Geometry check sheet. Reference: drawing and pictorial views, mm from the part's lowest x, y, z. A direction names the side the tool comes from. Round coordinates to 2 decimals unless told otherwise and drop trailing zeros. Order: outer loops, then holes, each group sorted by start corner. A loop starts at its lowest first (then second) coordinate and runs counter-clockwise, first axis right, second up. Notation, with made-up numbers: (77, 52) -> (105, 52) arc R16 cw to (105, 69) -> close; hole circle Ø5 at (-15, -11.5). An arc over 180 degrees is marked (long way). Return JSON: item names as keys, results as strings. Group by question number.
1) Draft check along Z on the marked faces 1, 2, 3 and 4. Enter one of: pulls with the +Z half, pulls with the -Z half, needs draft (parallel to the pull), parting line crosses it, or undercut.
2) Tool access check on the marked faces 5 and 6. Record the directions out of +Z, -Z, +X, -X, +Y, -Y that give a thin tool (end or side, any length) a straight path to the whole face; none if there is none.
3) Depth check by flat-ended pin: pin 1 (5 mm diameter, centred on x = 31, z = 24.5, fed in from +Y). Enter the tip coordinate at first touch or a pass-through.
4) Section check A-A on y = 22.25. Enter the section's corners in (x, z).
5) Section check C-C on z = 17. Enter the section's corners in (x, y), plus the area to 3 significant figures.
6) Section check B-B on x = 29. Enter the section's corners in (y, z).
7) Section check D-D on x = 12.5. Enter the section's corners in (y, z), plus the area to 3 significant figures.
8) Scan lines: L1, parallel to Z at x = 35, y = 5.75; L2, parallel to X at y = 21, z = 30; L3, parallel to Y at x = 31, z = 14. Record each from-to range of solid material in increasing order.
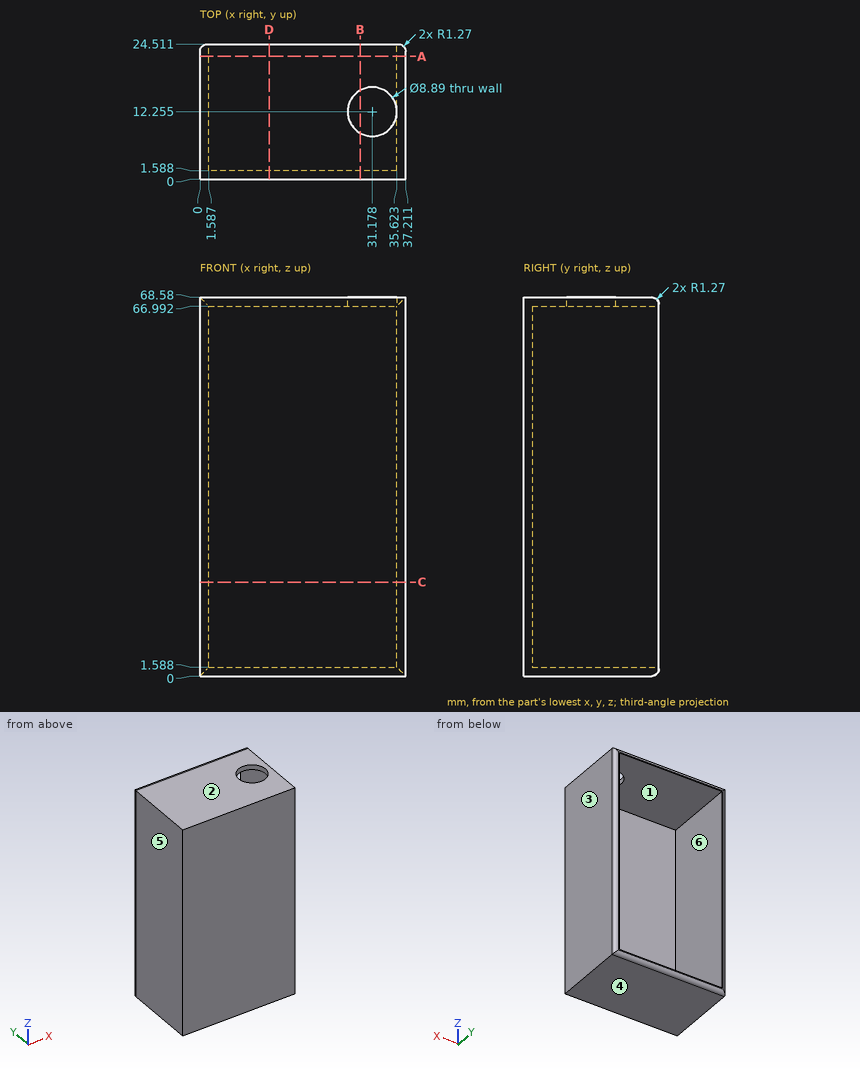
Check result:
{
 "1": {"face 1": "undercut", "face 2": "pulls with the +Z half", "face 3": "needs draft", "face 4": "pulls with the -Z half"},
 "2": {"face 5": "+Z, -Z, -X, +Y, -Y", "face 6": "+Y"},
 "3": {"pin 1": "y = 1.59"},
 "4": {"outline": "(0, 0) -> (37.21, 0) -> (37.21, 68.58) -> (0, 68.58) -> close; hole (1.59, 1.59) -> (35.62, 1.59) -> (35.62, 66.99) -> (1.59, 66.99) -> close"},
 "5": {"outline": "(0, 0) -> (37.21, 0) -> (37.21, 23.24) arc R1.27 ccw to (35.94, 24.51) -> (35.62, 24.51) -> (35.62, 1.59) -> (1.59, 1.59) -> (1.59, 24.51) -> (1.27, 24.51) arc R1.27 ccw to (0, 23.24) -> close", "area": "131 mm^2"},
 "6": {"outline": "(0, 0) -> (23.24, 0) arc R1.27 ccw to (24.51, 1.27) -> (24.51, 1.59) -> (1.59, 1.59) -> (1.59, 66.99) -> (8.38, 66.99) -> (8.38, 68.58) -> (0, 68.58) -> close; (16.13, 66.99) -> (24.51, 66.99) -> (24.51, 67.31) arc R1.27 ccw to (23.24, 68.58) -> (16.13, 68.58) -> close"},
 "7": {"outline": "(0, 0) -> (23.24, 0) arc R1.27 ccw to (24.51, 1.27) -> (24.51, 1.59) -> (1.59, 1.59) -> (1.59, 66.99) -> (24.51, 66.99) -> (24.51, 67.31) arc R1.27 ccw to (23.24, 68.58) -> (0, 68.58) -> close", "area": "181 mm^2"},
 "8": {"L1": "0 to 1.59, 66.99 to 68.58", "L2": "0 to 1.59, 35.62 to 37.21", "L3": "0 to 1.59"}
}
